For this review, take the finished solid that the model builds, in its own axes (mm). Face numbers are marked on the shaded views. A direction names the side the tool comes from. Round coordinates to 2 decimals unless told otherwise and drop trailing zeros. Loops run counter-clockwise (first coordinate to the right, second up) from the corner with the lowest first, then second, coordinate; pieces in that order, holes last. Notation, with made-up numbers: M 18.5,83 L 69.5,83 A15 cw 69.5,105 Z; hole C 78.5,-7.5 d9. An arc over 180 degrees is marked long. Write item = value, one per line. Start each with the question number.
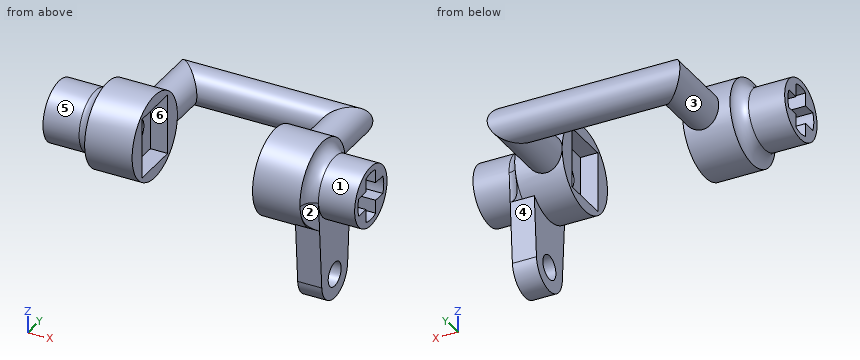
```python
from build123d import *

# Parameters (mm, degrees)
SWEEP_1_PROFILE_R        = 1.5
EXTRUDE_1_DEPTH          = 3.44
EXTRUDE_1_DEPTH_BACK     = 4.5
EXTRUDE_1_START          = 9.5
SKETCH_8_R               = 2.5
EXTRUDE_2_DEPTH          = 4.5
EXTRUDE_2_DEPTH_BACK     = 3.44
EXTRUDE_2_START          = -9.5
SKETCH_9_R               = 2.5
EXTRUDE_START            = 9.94
SKETCH_14_R              = 1
EXTRUDE_3_DEPTH          = 2
CUT_EXTRUDE_START        = 12.94
CUT_EXTRUDE_1_DEPTH      = 4
CUT_EXTRUDE_START_2      = -8.94
CUT_EXTRUDE_2_DEPTH      = 4
SKETCH_16_R              = 0.25
CUT_EXTRUDE_3_DEPTH      = 0.25
CUT_EXTRUDE_START_3      = 8.69
SKETCH_17_R              = 0.25
CUT_EXTRUDE_4_DEPTH      = 0.25
EXTRUDE_START_2          = 5
SKETCH_18_R              = 3.5
EXTRUDE_4_DEPTH          = 3.94
EXTRUDE_START_3          = -8.94
SKETCH_20_R              = 3.5
EXTRUDE_5_DEPTH          = 3.94
CUT_EXTRUDE_5_DEPTH      = 2
CUT_EXTRUDE_5_DEPTH_BACK = 2
SKETCH_22_W              = 1.44
SKETCH_22_H              = 5
CUT_EXTRUDE_6_DEPTH      = 19.653246417
CUT_EXTRUDE_6_DEPTH_BACK = 19.653246417
SKETCH_25_R              = 1
FILLET_1_R               = 1


with BuildPart() as part:
    # 扫描1: sweep along a path in 草图1
    with BuildLine(Plane.XY) as sweep_1_path:
        Line((9.5, 0), (6.5, 0))
        Line((6.5, 0), (6.5, 8))
        Line((6.5, 8), (-6.5, 8))
        Line((-6.5, 8), (-6.5, 0))
        Line((-6.5, 0), (-9.5, 0))
    # 扫描1 profile (on start of the path) → 扫描1 (sweep)
    with BuildSketch(Plane(origin=(9.5, 0, 0), x_dir=(0, -1, 0), z_dir=(-1, 0, 0))):
        Circle(SWEEP_1_PROFILE_R)
    sweep(path=sweep_1_path.line, transition=Transition.RIGHT)

    # 草图8 → 凸台-拉伸1 (add, two sides: drawn at the far end of the back side and taken through both)
    with BuildSketch(Plane(origin=(0, 0, 0), x_dir=(0, 0, -1), z_dir=(1, 0, 0)).offset(EXTRUDE_1_START - EXTRUDE_1_DEPTH_BACK)):
        with Locations(Location((0, 0, 0), (0, 0, 90))):
            Circle(SKETCH_8_R)
    extrude(amount=EXTRUDE_1_DEPTH + EXTRUDE_1_DEPTH_BACK)

    # 草图9 → 凸台-拉伸2 (add, two sides: drawn at the far end of the back side and taken through both)
    with BuildSketch(Plane(origin=(0, 0, 0), x_dir=(0, 0, -1), z_dir=(1, 0, 0)).offset(EXTRUDE_2_START - EXTRUDE_2_DEPTH_BACK)):
        with Locations(Location((0, 0, 0), (0, 0, 90))):
            Circle(SKETCH_9_R)
    extrude(amount=EXTRUDE_2_DEPTH + EXTRUDE_2_DEPTH_BACK)

    # 草图14 → 凸台-拉伸3 (add)
    with BuildSketch(Plane(origin=(0, 0, 0), x_dir=(0, 0, -1), z_dir=(1, 0, 0)).offset(EXTRUDE_START)):
        with BuildLine():
            Line((0.166666667, 2.494438258), (7.633333333, 1.995550606))
            ThreePointArc((7.633333333, 1.995550606), (9.5, 0), (7.633333333, -1.995550606))
            Line((7.633333333, -1.995550606), (0.166666667, -2.494438258))
            ThreePointArc((0.166666667, -2.494438258), (-2.5, 0), (0.166666667, 2.494438258))
        make_face()
        with Locations((7.5, 0)):
            Circle(SKETCH_14_R, mode=Mode.SUBTRACT)
    extrude(amount=-EXTRUDE_3_DEPTH)

    # 草图10 → 切除-拉伸1 (cut)
    with BuildSketch(Plane(origin=(0, 0, 0), x_dir=(0, 0, -1), z_dir=(1, 0, 0)).offset(CUT_EXTRUDE_START)):
        with BuildLine():
            Line((0.75, 0.75), (1.854049622, 0.75))
            ThreePointArc((1.854049622, 0.75), (2, 0), (1.854049622, -0.75))
            Line((1.854049622, -0.75), (0.75, -0.75))
            Line((0.75, -0.75), (0.75, -1.854049622))
            ThreePointArc((0.75, -1.854049622), (0, -2), (-0.75, -1.854049622))
            Line((-0.75, -1.854049622), (-0.75, -0.75))
            Line((-0.75, -0.75), (-1.854049622, -0.75))
            ThreePointArc((-1.854049622, -0.75), (-2, 0), (-1.854049622, 0.75))
            Line((-1.854049622, 0.75), (-0.75, 0.75))
            Line((-0.75, 0.75), (-0.75, 1.854049622))
            ThreePointArc((-0.75, 1.854049622), (0, 2), (0.75, 1.854049622))
            Line((0.75, 1.854049622), (0.75, 0.75))
        make_face()
    extrude(amount=-CUT_EXTRUDE_1_DEPTH, mode=Mode.SUBTRACT)

    # 草图11 → 切除-拉伸2 (cut)
    with BuildSketch(Plane(origin=(0, 0, 0), x_dir=(0, 0, -1), z_dir=(1, 0, 0)).offset(CUT_EXTRUDE_START_2)):
        with BuildLine():
            Line((0.75, 0.75), (0.75, 1.854049622))
            ThreePointArc((0.75, 1.854049622), (0, 2), (-0.75, 1.854049622))
            Line((-0.75, 1.854049622), (-0.75, 0.75))
            Line((-0.75, 0.75), (-1.854049622, 0.75))
            ThreePointArc((-1.854049622, 0.75), (-2, 0), (-1.854049622, -0.75))
            Line((-1.854049622, -0.75), (-0.75, -0.75))
            Line((-0.75, -0.75), (-0.75, -1.854049622))
            ThreePointArc((-0.75, -1.854049622), (0, -2), (0.75, -1.854049622))
            Line((0.75, -1.854049622), (0.75, -0.75))
            Line((0.75, -0.75), (1.854049622, -0.75))
            ThreePointArc((1.854049622, -0.75), (2, 0), (1.854049622, 0.75))
            Line((1.854049622, 0.75), (0.75, 0.75))
        make_face()
    extrude(amount=-CUT_EXTRUDE_2_DEPTH, mode=Mode.SUBTRACT)

    # 草图16 → 切除-拉伸3 (cut)
    with BuildSketch(Plane(origin=(0, 0, 0), x_dir=(0, 0, -1), z_dir=(1, 0, 0)).offset(CUT_EXTRUDE_START_2)):
        with Locations(Location((0.75, 0, 0), (0, 0, 90))):
            Circle(SKETCH_16_R)
    extrude(amount=CUT_EXTRUDE_3_DEPTH, mode=Mode.SUBTRACT)

    # 草图17 → 切除-拉伸4 (cut)
    with BuildSketch(Plane(origin=(0, 0, 0), x_dir=(0, 0, -1), z_dir=(1, 0, 0)).offset(CUT_EXTRUDE_START_3)):
        with Locations(Location((0.75, 0, 0), (0, 0, 90))):
            Circle(SKETCH_17_R)
    extrude(amount=CUT_EXTRUDE_4_DEPTH, mode=Mode.SUBTRACT)

    # 草图18 → 凸台-拉伸4 (add)
    with BuildSketch(Plane(origin=(0, 0, 0), x_dir=(0, 0, -1), z_dir=(1, 0, 0)).offset(EXTRUDE_START_2)):
        with Locations(Location((0, 0, 0), (0, 0, 90))):
            Circle(SKETCH_18_R)
    extrude(amount=EXTRUDE_4_DEPTH)

    # 草图20 → 凸台-拉伸5 (add)
    with BuildSketch(Plane(origin=(0, 0, 0), x_dir=(0, 0, -1), z_dir=(1, 0, 0)).offset(EXTRUDE_START_3)):
        with Locations(Location((0, 0, 0), (0, 0, 90))):
            Circle(SKETCH_20_R)
    extrude(amount=EXTRUDE_5_DEPTH)

    # 草图22 → 切除-拉伸5 (cut, two sides: drawn at the far end of the back side and taken through both)
    with BuildSketch(Plane(origin=(0, 0, 0), x_dir=(1, 0, 0), z_dir=(0, 1, 0)).offset(-CUT_EXTRUDE_5_DEPTH_BACK)):
        with Locations((-5.72, 0)):
            Rectangle(SKETCH_22_W, SKETCH_22_H)
        with Locations((5.72, 0)):
            Rectangle(SKETCH_22_W, SKETCH_22_H)
    extrude(amount=CUT_EXTRUDE_5_DEPTH + CUT_EXTRUDE_5_DEPTH_BACK, mode=Mode.SUBTRACT)

    # 草图25 → 切除-拉伸6 (cut, two sides: drawn at the far end of the back side and taken through both)
    with BuildSketch(Plane(origin=(0, 0, 0), x_dir=(0, 0, -1), z_dir=(1, 0, 0)).offset(-CUT_EXTRUDE_6_DEPTH_BACK)):
        Circle(SKETCH_25_R)
    extrude(amount=CUT_EXTRUDE_6_DEPTH + CUT_EXTRUDE_6_DEPTH_BACK, mode=Mode.SUBTRACT)

    # 圆角1
    # the kernel refuses this fillet: 1 mm, written as the material it adds along each edge
    with BuildSketch(Plane(origin=(-8.94, 0, 0), x_dir=(0, 1, 0), z_dir=(0, 0, 1))) as fillet_1_piece_1:
        with BuildLine():
            CenterArc((2.5 + FILLET_1_R, FILLET_1_R), FILLET_1_R, 180, 90)
            Line((2.5, FILLET_1_R), (2.5, 0))
            Line((2.5, 0), (2.5 + FILLET_1_R, 0))
        make_face()
    revolve(axis=Axis((-8.94, 0, 0), (-1, 0, 0)))
    with BuildSketch(Plane(origin=(8.94, 0, 0), x_dir=(0, 1, 0), z_dir=(0, 0, -1))) as fillet_1_piece_2:
        with BuildLine():
            CenterArc((2.5 + FILLET_1_R, FILLET_1_R), FILLET_1_R, 180, 90)
            Line((2.5 + FILLET_1_R, 0), (2.5, 0))
            Line((2.5, 0), (2.5, FILLET_1_R))
        make_face()
    revolve(axis=Axis((8.94, 0, 0), (1, 0, 0)), revolution_arc=183.822553729)
    with BuildSketch(Plane(origin=(8.94, -2.494438258, -0.166666667), x_dir=(1, 0, 0), z_dir=(0, 0.06666666666666658, -0.9977753031397177))) as fillet_1_piece_3_section:
        with BuildLine():
            CenterArc((FILLET_1_R, FILLET_1_R), FILLET_1_R, 180, 90)
            Line((0, FILLET_1_R), (0, 0))
            Line((0, 0), (FILLET_1_R, 0))
        make_face()
    fillet_1_piece_3 = extrude(amount=4.949489743, mode=Mode.PRIVATE)
    fillet_1_piece_3 = fillet_1_piece_3 & Plane(origin=(9.184299624, 0, 0), x_dir=(0, 1, 0), z_dir=(-1, 0, 0)) * Cylinder(3.5, 14, mode=Mode.PRIVATE)
    add(fillet_1_piece_3)
    with BuildSketch(Plane(origin=(8.94, 2.164472275, -5.105145295), x_dir=(0, 0.9977753031397177, -0.0666666666666666), z_dir=(0, 0.06666666666666658, 0.9977753031397177))) as fillet_1_piece_4_section:
        with BuildLine():
            CenterArc((FILLET_1_R, -FILLET_1_R), FILLET_1_R, 90, 90)
            Line((0, -FILLET_1_R), (0, 0))
            Line((0, 0), (FILLET_1_R, 0))
        make_face()
    fillet_1_piece_4 = extrude(amount=4.949489743, mode=Mode.PRIVATE)
    fillet_1_piece_4 = fillet_1_piece_4 & Plane(origin=(9.184299625, 0, 0), x_dir=(0, 1, 0), z_dir=(-1, 0, 0)) * Cylinder(3.5, 14, mode=Mode.PRIVATE)
    add(fillet_1_piece_4)
    with BuildSketch(Plane(origin=(8.94, 0, 0), x_dir=(0, 0.9977753030864385, -0.06666666746407793), z_dir=(0, -0.06666666746407793, -0.9977753030864385))) as fillet_1_piece_5:
        with BuildLine():
            CenterArc((2.5 + FILLET_1_R, FILLET_1_R), FILLET_1_R, 180, 90)
            Line((2.5, FILLET_1_R), (2.5, 0))
            Line((2.5, 0), (2.5 + FILLET_1_R, 0))
        make_face()
    revolve(axis=Axis((8.94, 0, 0), (1, 0, 0)), revolution_arc=3.822553775)


solid = part.part
```
(1) Draft analysis for pull direction Y (two halves, no side actions). For the marked faces 1, 2 and 3, state which applies: +Y half, -Y half, draft (parallel to the pull), parting line (faces both ways), or undercut.
(2) Add section C-C on y = 0. Count the separate pieces of the cut face and the enclosed holes in it, and give its area (3 significant figures).
(3) Wall thickness on L1, parallel to X at y = -2.75, z = 2; L2, parallel to X at y = 1.25, z = -1.5; L3, parallel to Y at x = 8.35, z = 0: over which ranges is each line inside the solid? List them lowest first.
(4) Add section D-D on x = 4.5. Write out the cut boundary in (y, z).
(5) Tool access review of the marked faces 4, 5 and 6: name each direction out of +Z, -Z, +X, -X, +Y, -Y from which nothing blocks a thin tool from reaching the whole face with its end or side.
(6) Add section A-A on x = 11. Write out the cut boundary in (y, z).
(7) For pin 1 Ø0.6 at (x, y) = (-11.5, 1) entering from +Z; pin 2 Ø1.4 at (y, z) = (-0.5, -7) entering from -X; pin 3 Ø1.5 at (y, z) = (0.5, -3.5) entering from +X; pin 4 Ø2 at (x, y) = (-1.5, 4) entering from -Z, all flat-tipped, find the tip position at first contact; note any pin that passes through.
(8) Add section B-B on y = 6. Write out the cut boundary in (x, z).
Answer sheet:
q1.face_1 = parting line
q1.face_2 = -Y half
q1.face_3 = undercut
q2.separate_pieces = 5
q2.enclosed_holes = 0
q2.area = 48.4 mm²
q3.L1 = -8.94 to -5, 5 to 8.94
q3.L2 = -12.94 to -6.44, 6.44 to 12.94
q3.L3 = -3.5 to -1, 1 to 3.5
q4.outline = C 8,0 d3
q5.face_4 = -Z, +X, -X, +Y
q5.face_5 = -X
q5.face_6 = none
q6.outline = C 0,0 d5; hole M -1.85,-0.75 L -0.75,-0.75 L -0.75,-1.85 A2 ccw 0.75,-1.85 L 0.75,-0.75 L 1.85,-0.75 A2 ccw 1.85,0.75 L 0.75,0.75 L 0.75,1.85 A2 ccw -0.75,1.85 L -0.75,0.75 L -1.85,0.75 A2 ccw Z
q7.pin_1 = 2.4
q7.pin_2 = 7.94
q7.pin_3 = 9.94
q7.pin_4 = through
q8.outline = C -6.5,0 d3; C 6.5,0 d3
